from build123d import *

# Parameters (mm, degrees)
CROQUIS1_R                       = 18.5
SALIENTE_EXTRUIR1_DEPTH          = 37
CROQUIS2_R                       = 6
CROQUIS2_R_2                     = 5
SALIENTE_EXTRUIR2_DEPTH          = 5
CROQUIS2_3_R                     = 3
SALIENTE_EXTRUIR3_DEPTH          = 20
TALADRO_DE_MARGEN_PARA_M31_D     = 3.4
TALADRO_DE_MARGEN_PARA_M31_DEPTH = 5


with BuildPart() as part:
    # Croquis1 → Saliente-Extruir1 (new body)
    with BuildSketch(Plane.XY):
        Circle(CROQUIS1_R)
    extrude(amount=SALIENTE_EXTRUIR1_DEPTH)

    # Croquis2 → Saliente-Extruir2 (add)
    with BuildSketch(Plane.XY.offset(37)):
        Circle(CROQUIS2_R)
        Circle(CROQUIS2_R_2, mode=Mode.SUBTRACT)
    extrude(amount=SALIENTE_EXTRUIR2_DEPTH)

    # Croquis2<3> → Saliente-Extruir3 (add)
    with BuildSketch(Plane.XY.offset(37)):
        Circle(CROQUIS2_3_R)
    extrude(amount=SALIENTE_EXTRUIR3_DEPTH)

    # Taladro de margen para M31
    with Locations(Plane(origin=(0, 0, 0), x_dir=(-1, 0, 0), z_dir=(0, 0, -1))):
        with Locations((0, 15.5), (13.423393759, 7.75), (13.423393759, -7.75), (0, -15.5), (-13.423393759, -7.75), (-13.423393759, 7.75)):
            Hole(TALADRO_DE_MARGEN_PARA_M31_D / 2, depth=TALADRO_DE_MARGEN_PARA_M31_DEPTH)


solid = part.part
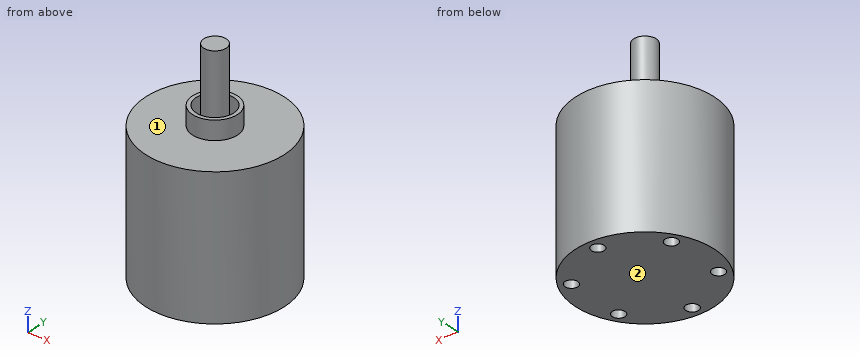
Geometry: final body of the model. Coordinates: model frame, mm. Face numbers are marked on the shaded views. A direction names the side the tool comes from. Round coordinates to 2 decimals unless told otherwise and drop trailing zeros. Order: outer loops, then holes, each group sorted by start corner. A loop starts at its lowest first (then second) coordinate and runs counter-clockwise, first axis right, second up. Notation, with made-up numbers: (75.25, 55) -> (83.25, 55) arc R21 ccw to (83.25, 93) -> close; hole circle Ø6 at (25, 39.25). An arc over 180 degrees is marked (long way). Put each result on its own line as item: value. Start each with the question number.
Q1. Reachability of the marked faces 1 and 2 from +Z, -Z, +X, -X, +Y, -Y: full face, straight path, thin tool, end or side. Return the list, or none.
Q2. Section B-B on z = 47.5. Return the cut outline in (x, y).
Q3. Section C-C on y = -1. Return the cut outline in (x, z), and give its area (3 significant figures).
Q4. First-contact query: pin 1 (5.5 mm diameter, centred on x = 13.42, y = 7.75, fed in from +Z); pin 2 (1 mm diameter, centred on x = 0.5, y = 15.5, fed in from -Z); pin 3 (10 mm diameter, centred on x = -1, z = 42.5, fed in from -Y). Flat tips, straight axial feed; report the tip coordinate or a pass-through.
Q5. Section D-D on x = 14. Return the cut outline in (y, z), and give its area (3 significant figures).
Q6. Line query: probe 1 along Y at (x, z) = (0, 1.45); probe 2 along Z at (x, y) = (-2, 17); probe 3 along Z at (x, y) = (0.5, 16). Output: solid intervals per line, ascending.
Q7. Section A-A on x = 0. Return the cut outline in (y, z), and give its area (4 significant figures).
Ans:
1. face 1: +Z
1. face 2: -Z, +X, -X, +Y, -Y
2. outline: circle Ø6 at (0, 0)
3. outline: (-18.47, 0) -> (18.47, 0) -> (18.47, 37) -> (5.92, 37) -> (5.92, 42) -> (4.9, 42) -> (4.9, 37) -> (2.83, 37) -> (2.83, 57) -> (-2.83, 57) -> (-2.83, 37) -> (-4.9, 37) -> (-4.9, 42) -> (-5.92, 42) -> (-5.92, 37) -> (-18.47, 37) -> close
3. area: 1,490 mm2
4. pin 1: stops at z = 37
4. pin 2: stops at z = 5
4. pin 3: stops at y = -6
5. outline: (-12.09, 0) -> (-9.35, 0) -> (-9.35, 5) -> (-6.15, 5) -> (-6.15, 0) -> (6.15, 0) -> (6.15, 5) -> (9.35, 5) -> (9.35, 0) -> (12.09, 0) -> (12.09, 37) -> (-12.09, 37) -> close
5. area: 863 mm2
6. probe 1: y = -18.5 to -17.2, -13.8 to 13.8, 17.2 to 18.5
6. probe 2: z = 0 to 37
6. probe 3: z = 5 to 37
7. outline: (-18.5, 0) -> (-17.2, 0) -> (-17.2, 5) -> (-13.8, 5) -> (-13.8, 0) -> (13.8, 0) -> (13.8, 5) -> (17.2, 5) -> (17.2, 0) -> (18.5, 0) -> (18.5, 37) -> (6, 37) -> (6, 42) -> (5, 42) -> (5, 37) -> (3, 37) -> (3, 57) -> (-3, 57) -> (-3, 37) -> (-5, 37) -> (-5, 42) -> (-6, 42) -> (-6, 37) -> (-18.5, 37) -> close
7. area: 1,465 mm2
